The model under review builds one solid part; all positions refer to its coordinate system, in mm. Face numbers are marked on the shaded views. Coordinates: 2 decimals unless noted, no trailing zeros. Write each loop counter-clockwise with the first axis right and the second up, starting at its lowest first coordinate (ties: lowest second). Pieces come first, ordered by that corner, then holes.
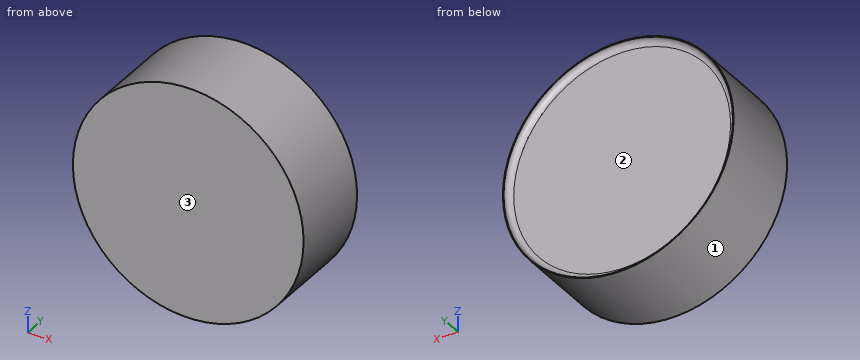
Autodesk Inventor part; units mm, degrees
ref_plane "YZ Plane" through (0, 0, 0) normal (1, 0, 0) x (0, 1, 0)
ref_plane "XZ Plane" through (0, 0, 0) normal (0, 1, 0) x (-1, 0, 0)
ref_plane "XY Plane" through (0, 0, 0) normal (0, 0, 1) x (1, 0, 0)
sketch "Sketch3" plane through (0, 0, 0) normal (0, 1, 0) x (-1, 0, 0)
  circle A0 centre (0, 0) radius 18.4
  dimension "d32" = 36.8
extrude "Extrusion4" add sketch "Sketch3" along normal blind 12.7
sketch "Sketch4" plane through (0, 12.7, 0) normal (0, 1, 0) x (1, 0, 0)
  circle A0 centre (0, 0) radius 18.4
  circle A1 centre (0, 0) radius 17.75
  circle A2 centre (0, 0) radius 18.4
  circle A3 centre (0, 0) radius 18.3
  dimension "d35" = 0.1
sketch "Sketch4 outline for Extrusion5" plane through (0, 12.7, 0) normal (0, 1, 0) x (1, 0, 0)
  circle A0 centre (0, 0) radius 18.4
  circle A1 centre (0, 0) radius 18.3
extrude "Extrusion5" add sketch "Sketch4 outline for Extrusion5" along normal blind 1
fillet "Fillet1" radius 1 1 edges at (-18.3, 12.7, 0)
equation "\"d32\" = icicles25D"
equation "\"d33\" = chairThickness"
equation "\"moduleHeight\" = 96"
equation "\"moduleMountD\" = 6.8"
equation "\"moduleCornerR\" = 5"
equation "\"d4\" = moduleCornerR"
equation "\"d5\" = moduleMountD"
equation "\"d6\" = moduleMountD"
equation "\"d8\" = moduleMountD"
equation "\"d10\" = moduleMountD"
equation "\"moduleOpeningR\" = 25"
equation "\"d13\" = moduleOpeningR"
equation "\"thickness\" = 6"
equation "\"d15\" = thickness"
equation "\"d16\" = 0"
equation "\"iciclesMountD\" = 42.5"
equation "\"d17\" = iciclesMountD"
equation "\"clearanceM3\" = 3.6"
equation "\"d18\" = clearanceM6"
equation "\"d21\" = 360deg"
equation "\"d0\" = moduleHeight"
equation "\"iciclesBaseOuterD\" = 48"
equation "\"iciclesPlugD\" = 35.5"
equation "\"chairThickness\" = 12.7"
equation "\"isiclesBaseThickness\" = 3"
equation "\"clearanceM6\" = 3.6"
equation "\"d7\" = iciclesBaseOuterD"
equation "\"d9\" = iciclesMountD"
equation "\"d22\" = 360deg"
equation "\"d24\" = isiclesBaseThickness"
equation "\"d25\" = 0"
equation "\"d29\" = isiclesBaseThickness"
equation "\"compressedGasket\" = 0.5"
equation "\"d31\" = 0"
equation "\"iciclesPlugNeck\" = 16"
equation "\"headClearanceM3\" = 5.6"
equation "\"d42\" = 360deg"
equation "\"d45\" = 0"
equation "\"iciclesFilletR\" = 2"
equation "\"d46\" = iciclesFilletR"
equation "\"d47\" = iciclesFilletR"
equation "\"icicles25D\" = 36.8"
equation "\"icicles25T\" = 8.4"
equation "\"icicles25ND\" = 18"
equation "\"insertM3\" = 4"
equation "\"d11\" = insertM3"
equation "\"isiclesPlugT\" = icicles25T"
equation "\"d30\" = isiclesPlugT + chairThickness + compressedGasket"
equation "\"d39\" = headClearanceM3"
properties part number "Module_bottom_Icicles26_v2_3DPrint"
Item 1: To check wall thickness, follow line 1 along Y through (x, z) = (-8, 7); line 2 along Z through (x, y) = (-2, 10); line 3 along Z through (x, y) = (-0.5, 2). State the ranges of each line that lie inside material, in increasing order.
Solved:
line 1: y = 0 to 12.7
line 2: z = -18.29 to 18.29
line 3: z = -18.39 to 18.39
Item 2: For pin 1 (1.5 mm diameter, centred on x = -6.5, y = 3, fed in from +Z); pin 2 (2 mm diameter, centred on x = -5.5, z = -9.5, fed in from +Y); pin 3 (1 mm diameter, centred on y = 10, z = 11.5, fed in from +X), all flat-tipped, find the tip position at first contact; note any pin that passes through.
Solved:
pin 1: stops at z = 17.48
pin 2: stops at y = 12.7
pin 3: stops at x = 14.75
Item 3: Take a section at A-A, the plane y = 7.25. Write out the cut boundary in (x, z).
Solved:
outline: circle Ø36.8 at (0, 0)
Item 4: Mouldability with a two-part tool opening along X and no side actions: class the marked faces 1, 2 and 3 as pulls with the +X half, pulls with the -X half, needs draft (parallel to the pull), parting line crosses it, or undercut.
Solved:
face 1: parting line crosses it
face 2: undercut
face 3: needs draft
